Verification items for this drawing (mm, ordinates from the low corner). Coordinates: 2 decimals unless noted, no trailing zeros. Order: outer loops, then holes, each group sorted by start corner. A loop starts at its lowest first (then second) coordinate and runs counter-clockwise, first axis right, second up.
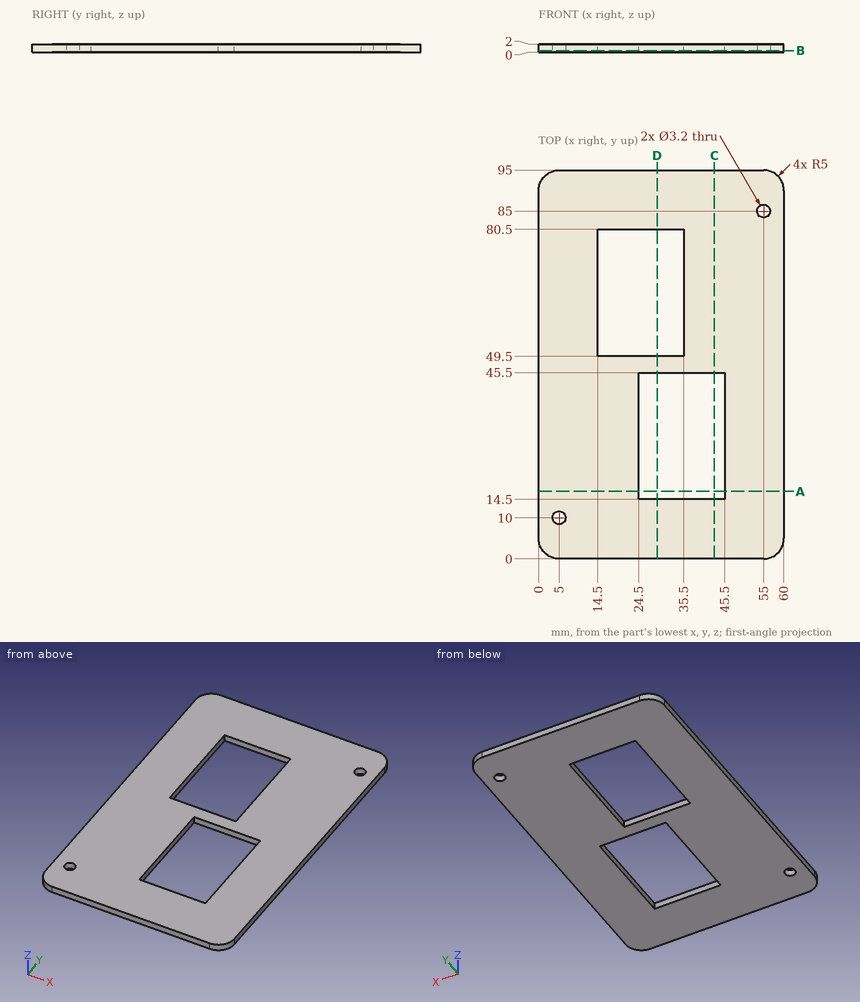
(1) Cross-section at B-B (z = 0.4). Enter the section's corners in (x, y), and give its area (3 significant figures).
Filled in:
outline: (0, 5) arc R5 ccw to (5, 0) - (55, 0) arc R5 ccw to (60, 5) - (60, 90) arc R5 ccw to (55, 95) - (5, 95) arc R5 ccw to (0, 90) - close; hole circle Ø3.2 at (5, 10); hole (14.5, 49.5) - (35.5, 49.5) - (35.5, 80.5) - (14.5, 80.5) - close; hole (24.5, 14.5) - (45.5, 14.5) - (45.5, 45.5) - (24.5, 45.5) - close; hole circle Ø3.2 at (55, 85)
area: 4,360 mm2
(2) Cross-section at D-D (x = 29). Enter the section's corners in (y, z), and give its area (3 significant figures).
Filled in:
outline: (0, 0) - (14.5, 0) - (14.5, 2) - (0, 2) - close; (45.5, 0) - (49.5, 0) - (49.5, 2) - (45.5, 2) - close; (80.5, 0) - (95, 0) - (95, 2) - (80.5, 2) - close
area: 66.0 mm2
(3) Cross-section at C-C (x = 43). Enter the section's corners in (y, z), and give its area (3 significant figures).
Filled in:
outline: (0, 0) - (14.5, 0) - (14.5, 2) - (0, 2) - close; (45.5, 0) - (95, 0) - (95, 2) - (45.5, 2) - close
area: 128 mm2
(4) Thickness scan on probe 1 along Y at (x, z) = (29, 0.95); probe 2 along X at (y, z) = (85, 0.75); probe 3 along Y at (x, z) = (55, 0.85). Record the ranges inside material, lowest first.
Filled in:
probe 1: y = 0 to 14.5, 45.5 to 49.5, 80.5 to 95
probe 2: x = 0 to 53.4, 56.6 to 60
probe 3: y = 0 to 83.4, 86.6 to 95
(5) Cross-section at A-A (y = 16.5). Enter the section's corners in (x, z), and give its area (3 significant figures).
Filled in:
outline: (0, 0) - (24.5, 0) - (24.5, 2) - (0, 2) - close; (45.5, 0) - (60, 0) - (60, 2) - (45.5, 2) - close
area: 78.0 mm2
